from build123d import *

# Parameters (mm, degrees)
CUT_EXTRUDE_START   = -4.02
SKETCH_2_R          = 1.67
CUT_EXTRUDE_1_DEPTH = 4.02


with BuildPart() as part:
    # 草图1 → 旋转1 (revolve)
    with BuildSketch(Plane.XY, mode=Mode.PRIVATE) as revolve_1_sk:
        Polygon((0, 0), (3.12, 0), (3.12, 5.36), (3.93, 5.36), (3.93, 6.14), (3.12, 6.14), (3.12, 8.24), (1.67, 8.24), (1.67, 12.16), (0, 12.16), align=None)
    revolve(revolve_1_sk.sketch.rotate(Axis((0, 0, 0), (0, 1, 0)), 90), axis=Axis((0, 0, 0), (0, 1, 0)))

    # 草图2 → 切除-拉伸1 (cut)
    with BuildSketch(Plane.XZ.offset(CUT_EXTRUDE_START)):
        with Locations(Location((0, 0, 0), (0, 0, 270))):
            Circle(SKETCH_2_R)
    extrude(amount=CUT_EXTRUDE_1_DEPTH, mode=Mode.SUBTRACT)

    # 草图3 → 切除-旋转1 (revolve, cut)
    with BuildSketch(Plane.XY, mode=Mode.PRIVATE) as cut_revolve_1_sk:
        Polygon((2.62, 0), (1.67, 0.95), (0, 0.95), (0, 0), align=None)
    revolve(cut_revolve_1_sk.sketch.rotate(Axis((0, 0, 0), (0, -1, 0)), 90), axis=Axis((0, 0, 0), (0, -1, 0)), mode=Mode.SUBTRACT)


solid = part.part
Here's how the part is built. I have some questions about the finished solid (model axes, mm). A direction names the side the tool comes from. Coordinates: 2 decimals unless noted, no trailing zeros. Order: outer loops, then holes, each group sorted by start corner. A loop starts at its lowest first (then second) coordinate and runs counter-clockwise, first axis right, second up.
Item 1: For P1, Ø2, axis at x = -2, z = -0.5, coming from the -Y side; P2, Ø2.5, axis at x = 0.5, z = 0, coming from the -Y side, each with a flat end and sliding along its axis, tell me the tip position at first contact or that it passes through.
Result sheet:
P1: stops at y = 0
P2: stops at y = 0.87
Item 2: I need wall thicknesses on line 1 (X direction, y = 1.85, z = 0); line 2 (Y direction, x = 3.5, z = 0.5); line 3 (Y direction, x = 0, z = -1.5). Which ranges of each line are inside material? Lowest first, please.
Result sheet:
line 1: x = -3.12 to -1.67, 1.67 to 3.12
line 2: y = 5.36 to 6.14
line 3: y = 4.02 to 12.16
Item 3: If we section it at C-C on y = 3.5: List the corners of the cut face in (x, z) for me, plus the area to 3 significant figures.
Result sheet:
outline: circle Ø6.24 at (0, 0); hole circle Ø3.34 at (0, 0)
area: 21.8 mm2
Item 4: If we mould it in two halves opening along Z, with no side actions, what happens to faces 4 (the face through (0, 12.16, 0)), 5 (the face through (0, 4.02, 0)), 6 (the face through (-0.937, 7.205, -2.976))? For each: +Z half, -Z half, draft (parallel to the pull), parting line (faces both ways), or undercut.
Result sheet:
face 4: draft
face 5: undercut
face 6: parting line
Item 5: If we section it at D-D on y = 7: List the corners of the cut face in (x, z) for me.
Result sheet:
outline: circle Ø6.24 at (0, 0)
Item 6: For faces 1 (the face through (-2, 6.14, 3)), 2 (the face through (-0.937, 2.718, -2.976)), 3 (the face through (-2, 0, -2)), which set-ups out of +Z, -Z, +X, -X, +Y, -Y let a thin tool reach every point of the face, with its end or its side?
Result sheet:
face 1: +Y
face 2: -Y
face 3: +Z, -Z, +X, -X, -Y
Item 7: If we section it at B-B on x = 0: List the corners of the cut face in (y, z) for me, plus the area to 3 significant figures.
Result sheet:
outline: (0, -3.12) - (5.36, -3.12) - (5.36, -3.93) - (6.14, -3.93) - (6.14, -3.12) - (8.24, -3.12) - (8.24, -1.67) - (12.16, -1.67) - (12.16, 1.67) - (8.24, 1.67) - (8.24, 3.12) - (6.14, 3.12) - (6.14, 3.93) - (5.36, 3.93) - (5.36, 3.12) - (0, 3.12) - (0, 2.62) - (0.95, 1.67) - (4.02, 1.67) - (4.02, -1.67) - (0.95, -1.67) - (0, -2.62) - close
area: 51.4 mm2
Item 8: If we section it at A-A on z = 0: List the corners of the cut face in (x, y) for me, plus the area to 3 significant figures.
Result sheet:
outline: (-3.93, 5.36) - (-3.12, 5.36) - (-3.12, 0) - (-2.62, 0) - (-1.67, 0.95) - (-1.67, 4.02) - (1.67, 4.02) - (1.67, 0.95) - (2.62, 0) - (3.12, 0) - (3.12, 5.36) - (3.93, 5.36) - (3.93, 6.14) - (3.12, 6.14) - (3.12, 8.24) - (1.67, 8.24) - (1.67, 12.16) - (-1.67, 12.16) - (-1.67, 8.24) - (-3.12, 8.24) - (-3.12, 6.14) - (-3.93, 6.14) - close
area: 51.4 mm2
